Print and shaded views of the part. All mm, measured from the part's lowest x, y and z. A direction names the side the tool comes from. Round coordinates to 2 decimals unless told otherwise and drop trailing zeros. Write each loop counter-clockwise with the first axis right and the second up, starting at its lowest first coordinate (ties: lowest second). Pieces come first, ordered by that corner, then holes.
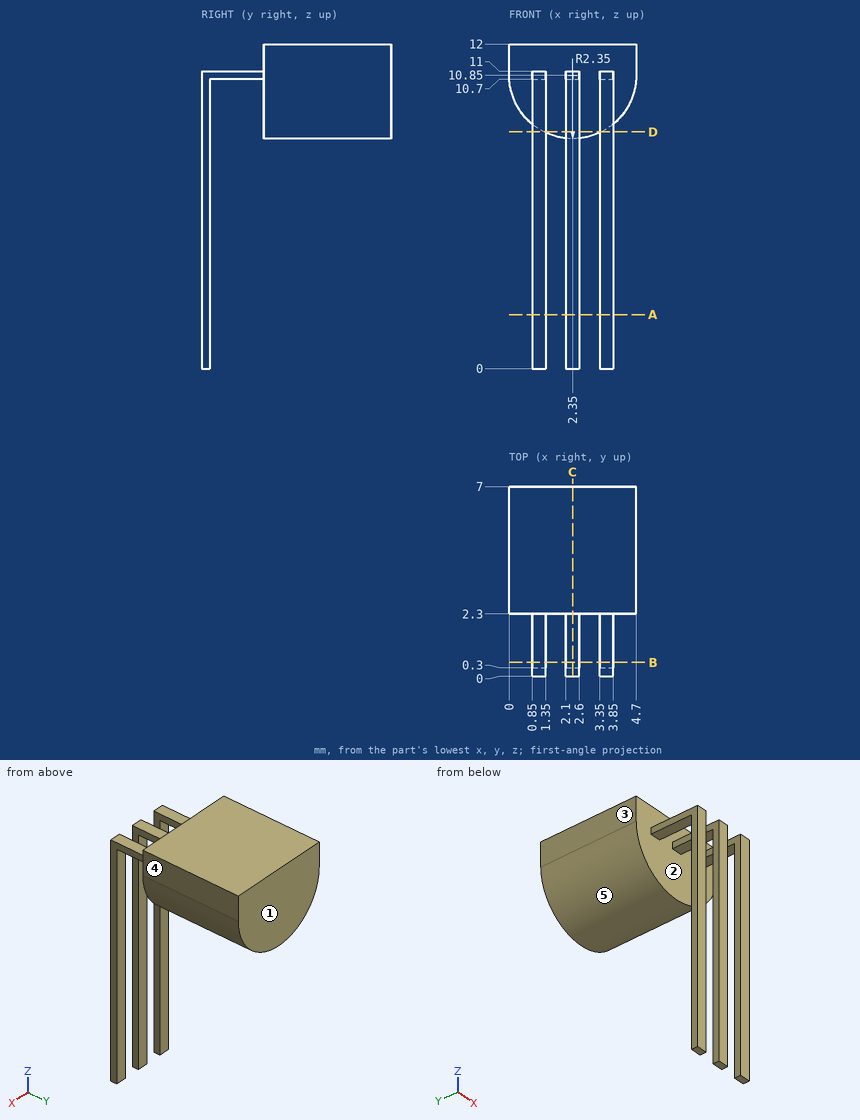
1) Wall check: L1, parallel to Y at x = 2.45, z = 9.5; L2, parallel to Y at x = 3.1, z = 10.25; L3, parallel to Y at x = 1.1, z = 5.5. Give the ranges that are in metal, low to high.
Results:
L1: y = 0 to 0.3, 2.3 to 7
L2: y = 2.3 to 7
L3: y = 0 to 0.3
2) Slice it at D-D (z = 8.75). Write the cut outline in (x, y).
Results:
outline: (0.85, 0) - (1.35, 0) - (1.35, 0.3) - (0.85, 0.3) - close; (1.3, 2.3) - (3.4, 2.3) - (3.4, 7) - (1.3, 7) - close; (2.1, 0) - (2.6, 0) - (2.6, 0.3) - (2.1, 0.3) - close; (3.35, 0) - (3.85, 0) - (3.85, 0.3) - (3.35, 0.3) - close
3) Slice it at A-A (z = 2). Write the cut outline in (x, y), plus the area to 3 significant figures.
Results:
outline: (0.85, 0) - (1.35, 0) - (1.35, 0.3) - (0.85, 0.3) - close; (2.1, 0) - (2.6, 0) - (2.6, 0.3) - (2.1, 0.3) - close; (3.35, 0) - (3.85, 0) - (3.85, 0.3) - (3.35, 0.3) - close
area: 0.450 mm2
4) Slice it at B-B (y = 0.5). Write the cut outline in (x, z).
Results:
outline: (0.85, 10.7) - (1.35, 10.7) - (1.35, 11) - (0.85, 11) - close; (2.1, 10.7) - (2.6, 10.7) - (2.6, 11) - (2.1, 11) - close; (3.35, 10.7) - (3.85, 10.7) - (3.85, 11) - (3.35, 11) - close
5) Slice it at C-C (x = 2.35). Write the cut outline in (y, z).
Results:
outline: (0, 0) - (0.3, 0) - (0.3, 10.7) - (2.3, 10.7) - (2.3, 8.5) - (7, 8.5) - (7, 12) - (2.3, 12) - (2.3, 11) - (0, 11) - close
6) Mould opens along Y. For the marked faces 1, 2 and 3 say: released by +Y, released by -Y, zero draft, split by the parting line, or undercut.
Results:
face 1: released by +Y
face 2: undercut
face 3: zero draft
7) Which spindle directions (+Z, -Z, +X, -X, +Y, -Y) get a long thin tool onto all of the face, cutting with end or side? Do the marked faces 4 and 5. Say none if no direction does.
Results:
face 4: +Z, -Z, +X, +Y, -Y
face 5: -Z, +Y
8) Pin check, flat tips, straight feed: pin 1 Ø1 at (x, z) = (2.5, 9.5) entering from -Y; pin 2 Ø1.2 at (y, z) = (1, 6.5) entering from -X; pin 3 Ø0.7 at (y, z) = (0.5, 4.5) entering from +X; pin 4 Ø0.6 at (x, z) = (2.5, 3.5) entering from +Y. Stop position of each tip, or through.
Results:
pin 1: stops at y = 0
pin 2: passes through
pin 3: stops at x = 3.85
pin 4: stops at y = 0.3
